```python
from build123d import *

# Parameters (mm, degrees)
F0_W     = 150
F0_H     = 30
F1_DEPTH = 80
F3_DEPTH = 20
F4_DEPTH = 10
F5_R     = 5
F7_DEPTH = 20
F8_DEPTH = 10


with BuildPart() as f1:
    # F0 (on Top) → F1 (new body)
    with BuildSketch(Plane.XY):
        Rectangle(F0_W, F0_H)
    extrude(amount=F1_DEPTH)

    # F2 (on face) → F3 (join)
    with BuildSketch(Plane.XZ.offset(15)):
        with BuildLine():
            ThreePointArc((5, 20.635083), (15.811388, 27.752551), (20, 40))
            ThreePointArc((20, 40), (15.811388, 52.247449), (5, 59.364917))
            Line((5, 59.364917), (5, 50))
            Line((5, 50), (0, 50))
            Line((0, 50), (-5, 50))
            Line((-5, 50), (-5, 59.364917))
            ThreePointArc((-5, 59.364917), (-20, 40), (-5, 20.635083))
            Line((-5, 20.635083), (-5, 30))
            Line((-5, 30), (0, 30))
            Line((0, 30), (5, 30))
            Line((5, 30), (5, 20.635083))
        make_face()
    extrude(amount=F3_DEPTH)

    # F2 (on face) → F4 (join)
    with BuildSketch(Plane.XZ.offset(15)):
        with BuildLine():
            Line((5, 50), (5, 59.364917))
            ThreePointArc((5, 59.364917), (2.520086, 59.840594), (0, 60))
            Line((0, 60), (0, 50))
            Line((0, 50), (5, 50))
        make_face()
        with BuildLine():
            Line((0, 50), (0, 60))
            ThreePointArc((0, 60), (-2.520086, 59.840594), (-5, 59.364917))
            Line((-5, 59.364917), (-5, 50))
            Line((-5, 50), (0, 50))
        make_face()
        with BuildLine():
            ThreePointArc((0, 20), (2.520086, 20.159406), (5, 20.635083))
            Line((5, 20.635083), (5, 30))
            Line((5, 30), (0, 30))
            Line((0, 30), (0, 20))
        make_face()
        with BuildLine():
            ThreePointArc((-5, 20.635083), (-2.520086, 20.159406), (0, 20))
            Line((0, 20), (0, 30))
            Line((0, 30), (-5, 30))
            Line((-5, 30), (-5, 20.635083))
        make_face()
    extrude(amount=F4_DEPTH)

    # F5
    f5_edges = [f1.edges().sort_by_distance(p)[0] for p in [
        (0, -15, 80),
        (0, 15, 80),
        (0, -15, 0),
        (0, 15, 0),
        (75, -15, 40),
        (75, 15, 40),
        (-75, -15, 40),
        (-75, 15, 40),
    ]]
    fillet(f5_edges, radius=F5_R)

    # F6 (on face) → F7 (cut)
    with BuildSketch(Plane(origin=(0, 15, 0), x_dir=(-1, 0, 0), z_dir=(0, 1, 0))):
        with BuildLine():
            ThreePointArc((5, 20.635083), (15.811388, 27.752551), (20, 40))
            ThreePointArc((20, 40), (15.811388, 52.247449), (5, 59.364917))
            Line((5, 59.364917), (5, 50))
            Line((5, 50), (0, 50))
            Line((0, 50), (-5, 50))
            Line((-5, 50), (-5, 59.364917))
            ThreePointArc((-5, 59.364917), (-20, 40), (-5, 20.635083))
            Line((-5, 20.635083), (-5, 30))
            Line((-5, 30), (0, 30))
            Line((0, 30), (5, 30))
            Line((5, 30), (5, 20.635083))
        make_face()
    extrude(amount=-F7_DEPTH, mode=Mode.SUBTRACT)

    # F6 (on face) → F8 (cut)
    with BuildSketch(Plane(origin=(0, 15, 0), x_dir=(-1, 0, 0), z_dir=(0, 1, 0))):
        with BuildLine():
            Line((5, 50), (5, 59.364917))
            ThreePointArc((5, 59.364917), (2.520086, 59.840594), (0, 60))
            Line((0, 60), (0, 50))
            Line((0, 50), (5, 50))
        make_face()
        with BuildLine():
            Line((0, 50), (0, 60))
            ThreePointArc((0, 60), (-2.520086, 59.840594), (-5, 59.364917))
            Line((-5, 59.364917), (-5, 50))
            Line((-5, 50), (0, 50))
        make_face()
        with BuildLine():
            ThreePointArc((0, 20), (2.520086, 20.159406), (5, 20.635083))
            Line((5, 20.635083), (5, 30))
            Line((5, 30), (0, 30))
            Line((0, 30), (0, 20))
        make_face()
        with BuildLine():
            ThreePointArc((-5, 20.635083), (-2.520086, 20.159406), (0, 20))
            Line((0, 20), (0, 30))
            Line((0, 30), (-5, 30))
            Line((-5, 30), (-5, 20.635083))
        make_face()
    extrude(amount=-F8_DEPTH, mode=Mode.SUBTRACT)


solid = f1.part
```
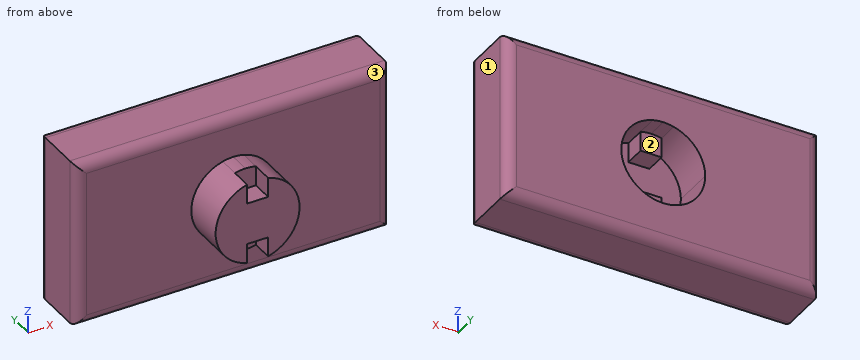
Work out the finished part from the listing and answer in its coordinate system (mm). Face numbers are marked on the shaded views. Round coordinates to 2 decimals unless told otherwise and drop trailing zeros. Order: outer loops, then holes, each group sorted by start corner. A loop starts at its lowest first (then second) coordinate and runs counter-clockwise, first axis right, second up.
Q1. Given pin 1 Ø5 at (x, y) = (-12, -27) entering from +Z; pin 2 Ø3 at (y, z) = (-32.5, 23) entering from -X; pin 3 Ø3 at (x, y) = (4.5, -16) entering from -Z, each flat-ended and moving along its own axis, determine where each tip first touches the part or whether it passes through.
Solution:
pin 1: stops at z = 57.6
pin 2: stops at x = -12.64
pin 3: stops at z = 2.82
Q2. A cutting plane is placed at A-A, the plane y = 0. Determine the outline of the cut face in (x, z), then the cut area to 3 significant figures.
Solution:
outline: (-75, 0) - (75, 0) - (75, 80) - (-75, 80) - close; hole (-5, 20.64) - (-5, 30) - (5, 30) - (5, 20.64) arc R20 ccw to (5, 59.36) - (5, 50) - (-5, 50) - (-5, 59.36) arc R20 ccw to start
area: 10,900 mm2
Q3. A cutting plane is placed at C-C, the plane y = -19.5. Determine the outline of the cut face in (x, z), then the cut area to 3 significant figures.
Solution:
outline: (-5, 20.64) arc R20 ccw to (5, 20.64) arc R20 ccw to (5, 59.36) arc R20 ccw to (-5, 59.36) arc R20 ccw to start
area: 1,260 mm2
Q4. The mould has two halves that part along X. Classify the marked faces 1, 2 and 3: pulls with the +X half, pulls with the -X half, needs draft (parallel to the pull), parting line crosses it, or undercut.
Solution:
face 1: pulls with the +X half
face 2: undercut
face 3: needs draft
Q5. Find the intervals of material crossed by line 1 along Y through (x, z) = (58, 46.5); line 2 along Y through (x, z) = (4, 52.5); line 3 along X through (y, z) = (9, 36), in increasing order.
Solution:
line 1: y = -15 to 15
line 2: y = -25 to 5
line 3: x = -75 to -19.6, 19.6 to 75
Q6. A cutting plane is placed at B-B, the plane x = -59. Determine the outline of the cut face in (y, z), then the cut area to 3 significant figures.
Solution:
outline: (-15, 5) arc R5 ccw to (-10, 0) - (10, 0) arc R5 ccw to (15, 5) - (15, 75) arc R5 ccw to (10, 80) - (-10, 80) arc R5 ccw to (-15, 75) - close
area: 2,380 mm2
Q7. A cutting plane is placed at D-D, the plane z = 31.5. Determine the outline of the cut face in (x, y), then the cut area to 3 significant figures.
Solution:
outline: (-75, -10) arc R5 ccw to (-70, -15) - (-18.1, -15) - (-18.1, -35) - (18.1, -35) - (18.1, -15) - (70, -15) arc R5 ccw to (75, -10) - (75, 10) arc R5 ccw to (70, 15) - (18.1, 15) - (18.1, -5) - (-18.1, -5) - (-18.1, 15) - (-70, 15) arc R5 ccw to (-75, 10) - close
area: 4,480 mm2
